from build123d import *

# Parameters (mm, degrees)
SKETCH1_R                  = 2.25
SKETCH1_R_2                = 1.725
BASE_FLANGE1_DEPTH         = 1.5748
SKETCHED_START             = 0.25
SKETCHED_BEND1_OUTLINE_W   = 50
SKETCHED_BEND1_OUTLINE_H   = 1.5748
SKETCHED_BEND1_DEPTH       = 78.867027748
SKETCHED_START_2           = 78.810179492
SKETCHED_BEND1_2_OUTLINE_R = 2.25
SKETCHED_BEND1_2_DEPTH     = 3.2512
SKETCHED_START_3           = -39
SKETCHED_BEND1_3_DEPTH     = 78


with BuildPart() as part:
    # Base-Flange1: sheet metal written as solids
    # Sketch1 → Base-Flange1 (new body)
    with BuildSketch(Plane.XY):
        with BuildLine():
            Line((0.25, 38.499188303), (0.25, 26.248809497))
            ThreePointArc((0.25, 26.248809497), (26.498809497, 0), (0.25, -26.248809497))
            Line((0.25, -26.248809497), (0.25, -38.499188303))
            ThreePointArc((0.25, -38.499188303), (16.257038834, -34.95934997), (29.278831944, -25))
            Line((29.278831944, -25), (80.25, -25))
            Line((80.25, -25), (105.25, -25))
            Line((105.25, -25), (105.25, 25))
            Line((105.25, 25), (80.25, 25))
            Line((80.25, 25), (29.278831944, 25))
            ThreePointArc((29.278831944, 25), (16.257038834, 34.95934997), (0.25, 38.499188303))
        make_face()
        with Locations((12.819894984, 30.949964339)):
            Circle(SKETCH1_R, mode=Mode.SUBTRACT)
        with Locations((30.949964339, 12.819894984)):
            Circle(SKETCH1_R, mode=Mode.SUBTRACT)
        with Locations((30.949964339, -12.819894984)):
            Circle(SKETCH1_R, mode=Mode.SUBTRACT)
        with Locations((12.819894984, -30.949964339)):
            Circle(SKETCH1_R, mode=Mode.SUBTRACT)
        with Locations((100.25, 20)):
            Circle(SKETCH1_R_2, mode=Mode.SUBTRACT)
        with Locations((85.25, 20)):
            Circle(SKETCH1_R_2, mode=Mode.SUBTRACT)
        with Locations((85.25, -20)):
            Circle(SKETCH1_R_2, mode=Mode.SUBTRACT)
        with Locations((100.25, -20)):
            Circle(SKETCH1_R_2, mode=Mode.SUBTRACT)
    extrude(amount=-BASE_FLANGE1_DEPTH)

    # Sketched Bend1: read off the stored shape, not the designer's step
    # Sketched Bend1 outline → Sketched Bend1 (cut)
    with BuildSketch(Plane.YZ.offset(SKETCHED_START)):
        with Locations((0, -0.7874)):
            Rectangle(SKETCHED_BEND1_OUTLINE_W, SKETCHED_BEND1_OUTLINE_H)
    extrude(amount=SKETCHED_BEND1_DEPTH, mode=Mode.SUBTRACT)

    # Sketched Bend1 2 outline → Sketched Bend1 2 (add)
    with BuildSketch(Plane.YZ.offset(SKETCHED_START_2)):
        with BuildLine():
            Line((25, 0), (25, 50.836188564))
            ThreePointArc((25, 50.836188564), (34.95934997, 63.857981674), (38.499188303, 79.865020508))
            Line((38.499188303, 79.865020508), (26.248809497, 79.865020508))
            ThreePointArc((26.248809497, 79.865020508), (0, 53.616211011), (-26.248809497, 79.865020508))
            Line((-26.248809497, 79.865020508), (-38.499188303, 79.865020508))
            ThreePointArc((-38.499188303, 79.865020508), (-34.95934997, 63.857981674), (-25, 50.836188564))
            Line((-25, 50.836188564), (-25, 0))
            Line((-25, 0), (25, 0))
        make_face()
        with Locations((-12.819894984, 49.165056169)):
            Circle(SKETCHED_BEND1_2_OUTLINE_R, mode=Mode.SUBTRACT)
        with Locations((-30.949964339, 67.295125524)):
            Circle(SKETCHED_BEND1_2_OUTLINE_R, mode=Mode.SUBTRACT)
        with Locations((12.819894984, 49.165056169)):
            Circle(SKETCHED_BEND1_2_OUTLINE_R, mode=Mode.SUBTRACT)
        with Locations((30.949964339, 67.295125524)):
            Circle(SKETCHED_BEND1_2_OUTLINE_R, mode=Mode.SUBTRACT)
    extrude(amount=SKETCHED_BEND1_2_DEPTH)

    # Sketched Bend1 3 outline → Sketched Bend1 3 (cut)
    with BuildSketch(Plane(origin=(0, 0, 0), x_dir=(1, 0, 0), z_dir=(0, 1, 0)).offset(SKETCHED_START_3)):
        with BuildLine():
            ThreePointArc((82.061379492, 0), (80.875985684, -0.491006192), (80.384979492, -1.6764))
            Line((80.384979492, -1.6764), (80.384979492, -79.865020508))
            Line((80.384979492, -79.865020508), (82.061379492, -79.865020508))
            Line((82.061379492, -79.865020508), (82.061379492, 0))
        make_face()
        with BuildLine():
            Line((78.810179493, -81), (78.810179492, -1.6764))
            ThreePointArc((78.810179492, -1.6764), (79.762433925, 0.622545567), (82.061379492, 1.5748))
            Line((82.061379492, 1.5748), (84, 1.5748))
            Line((84, 1.5748), (84, 3))
            Line((84, 3), (-1, 3))
            Line((-1, 3), (-1, -81))
            Line((-1, -81), (78.810179493, -81))
        make_face()
    extrude(amount=SKETCHED_BEND1_3_DEPTH, mode=Mode.SUBTRACT)


solid = part.part
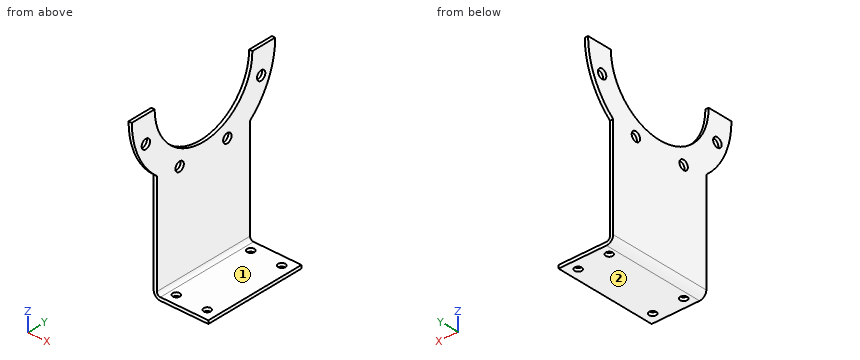
Input: part model. Units: mm. Frame: model coordinates. Face numbers are marked on the shaded views. A direction names the side the tool comes from. Round coordinates to 2 decimals unless told otherwise and drop trailing zeros. Order: outer loops, then holes, each group sorted by start corner. A loop starts at its lowest first (then second) coordinate and runs counter-clockwise, first axis right, second up. Notation, with made-up numbers: (36.5, -16) - (42.5, -16) arc R22 cw to (42.5, 19) - close; hole circle Ø2 at (8, -21). An arc over 180 degrees is marked (long way). Answer as a JSON object with one key per item and string values. Group by question number.
(1) Material intervals for probe 1 along Y at (x, z) = (85.25, -0.55) (3 decimals); probe 2 along X at (y, z) = (-6, 15.5); probe 3 along Z at (x, y) = (83.5, 18), sorted ascending. Write a range as from..to.
(2) Cut plane B-B (y = -20). Return loops of the section in (x, z) (3 decimals), then the cut area to 3 significant figures.
(3) Cut plane A-A (x = 85.25). Return loops of the section in (y, z) (3 decimals).
(4) Cut plane C-C (z = 57.5). Return loops of the section in (x, y), then the cut area to 3 significant figures.
(5) Pin query (flat end, axial travel): P1, Ø3.5, axis at y = -12.82, z = 49.17, coming from the -X side; P2, Ø11.5, axis at x = 96, y = 4.5, coming from the +Z side; P3, Ø7, axis at y = 12.82, z = 49.17, coming from the +X side (3 decimals). Return the tip coordinate at first contact, or that it passes through.
(6) Reachability of the marked faces 1 and 2 from +Z, -Z, +X, -X, +Y, -Y: full face, straight path, thin tool, end or side. Return the list, or none.
(7) Cut plane D-D (y = 0). Return loops of the section in (x, z), then the cut area to 3 significant figures.
Here are the results:
{
 "1": {"probe 1": "y = -25..-21.725, -18.275..18.275, 21.725..25", "probe 2": "x = 78.81..80.38", "probe 3": "z = -1.57..0"},
 "2": {"outline": "(78.81, 1.676) arc R3.251 ccw to (82.061, -1.575) - (83.525, -1.575) - (83.525, 0) - (82.061, 0) arc R1.676 cw to (80.385, 1.676) - (80.385, 62.865) - (78.81, 62.865) - close; (86.975, -1.575) - (98.525, -1.575) - (98.525, 0) - (86.975, 0) - close; (101.975, -1.575) - (105.25, -1.575) - (105.25, 0) - (101.975, 0) - close", "area": "128 mm^2"},
 "3": {"outline": "(-25, -1.575) - (-21.725, -1.575) - (-21.725, 0) - (-25, 0) - close; (-18.275, -1.575) - (18.275, -1.575) - (18.275, 0) - (-18.275, 0) - close; (21.725, -1.575) - (25, -1.575) - (25, 0) - (21.725, 0) - close"},
 "4": {"outline": "(78.81, -31.21) - (80.38, -31.21) - (80.38, -13.74) - (78.81, -13.74) - close; (78.81, 13.74) - (80.38, 13.74) - (80.38, 31.21) - (78.81, 31.21) - close", "area": "55.0 mm^2"},
 "5": {"P1": "passes through", "P2": "stops at z = 0", "P3": "stops at x = 80.385"},
 "6": {"face 1": "+Z, +X, +Y, -Y", "face 2": "-Z, +X, -X, +Y, -Y"},
 "7": {"outline": "(78.81, 1.68) arc R3.25 ccw to (82.06, -1.57) - (105.25, -1.57) - (105.25, 0) - (82.06, 0) arc R1.68 cw to (80.38, 1.68) - (80.38, 53.62) - (78.81, 53.62) - close", "area": "124 mm^2"}
}
